The model under review builds one solid part; all positions refer to its coordinate system, in mm. A direction names the side the tool comes from. Coordinates: 2 decimals unless noted, no trailing zeros. Write each loop counter-clockwise with the first axis right and the second up, starting at its lowest first coordinate (ties: lowest second). Pieces come first, ordered by that corner, then holes. Notation, with made-up numbers: (-2.5, 64.5) - (2.5, 64.5) arc R25 cw to (2.5, 84.5) - close; hole circle Ø1 at (73, 14.25). An arc over 180 degrees is marked (long way). Return JSON: item names as keys, results as strings. Group by question number.
(1) We need section A-A on z = 220.5. State the section outline as (x, y) points.
(2) We need section C-C on x = -3.5. Give the number of separate pieces and of enclosed holes in the cut face, then the cut area to 3 significant figures.
(3) Draft analysis for pull direction Z (two halves, no side actions). For faces 5 (the face through (4.65, 9.8, 213.87)), 6 (the face through (-6, 4, 260.5)), 7 (the face through (-5, 4, 205.5)), state which applies: released by +Z, released by -Z, zero draft, split by the parting line, or undercut.
(4) To check wall thickness, follow L1, parallel to X at y = 1, z = 208.5; L2, parallel to Z at x = -3.5, y = 2.5; L3, parallel to X at y = 5, z = 223.5. State the ranges of each line that lie inside material, in increasing order. Write a range as from..to.
(5) Tool access review of faces 1 (the face through (-15.93, 9.8, 213.85)), 2 (the face through (4.65, -2.8, 213.87)), 3 (the face through (10, 4, 253)), 4 (the face through (-16.3, 4, 233)): name each direction out of +Z, -Z, +X, -X, +Y, -Y from which nothing blocks a thin tool from reaching the whole face with its end or side.
(6) We need section B-B on y = 5.75. State the section outline as (x, z) points.
(7) We need section D-D on x = -10.5. State the section outline as (y, z) points, then the cut area to 3 significant figures.
(8) For pin 1 Ø1 at (y, z) = (0, 246) entering from +X; pin 2 Ø3.5 at (y, z) = (4, 255) entering from +X; pin 3 Ø2.5 at (x, z) = (-3.5, 208.5) entering from +Y; pin 4 Ø5 at (x, z) = (-16.5, 257.5) entering from +Y, all flat-tipped, find the tip position at first contact; note any pin that passes through.
```python
from build123d import *

# Parameters (mm, degrees)
SKETCH151_R     = 1.6
PAD085_DEPTH    = 13
CHAMFER055_SIZE = 1
FILLET050_R     = 5
CHAMFER061_SIZE = 0.4


with BuildPart() as part:
    # Sketch151 → Pad085 (new body)
    with BuildSketch(Plane.XZ):
        with BuildLine():
            Line((-11.3, 27.5), (20, 27.5))
            Line((20, 11.599342), (20, 27.5))
            ThreePointArc((20, -3.599342), (25.5, 4), (20, 11.599342))
            Line((20, -27.5), (20, -3.599342))
            Line((20, -27.5), (-11.3, -27.5))
            Line((-11.3, -27.5), (-11.3, 27.5))
        make_face()
        with Locations((-6.5, 24.5)):
            Circle(SKETCH151_R, mode=Mode.SUBTRACT)
        with Locations((6.5, 24.5)):
            Circle(SKETCH151_R, mode=Mode.SUBTRACT)
        with Locations((-6.5, -24.5)):
            Circle(SKETCH151_R, mode=Mode.SUBTRACT)
        with Locations((6.5, -24.5)):
            Circle(SKETCH151_R, mode=Mode.SUBTRACT)
        with BuildLine():
            Line((-6.3, 19.5), (15, 19.5))
            Line((15, 8.330127), (15, 19.5))
            ThreePointArc((15, -0.330127), (22.5, 4), (15, 8.330127))
            Line((15, -19.5), (15, -0.330127))
            Line((15, -19.5), (-6.3, -19.5))
            Line((-6.3, -19.5), (-6.3, 19.5))
        make_face(mode=Mode.SUBTRACT)
    extrude(amount=PAD085_DEPTH)

    # Chamfer055
    chamfer055_edges = [part.edges().sort_by_distance(p)[0] for p in [
        (-11.3, -6.5, -27.5),
        (20, -6.5, -27.5),
        (-11.3, -6.5, 27.5),
        (20, -6.5, 27.5),
        (-6.3, -6.5, 19.5),
        (-6.3, -6.5, -19.5),
        (15, -6.5, -19.5),
        (15, -6.5, 19.5),
    ]]
    chamfer(chamfer055_edges, length=CHAMFER055_SIZE)

    # Fillet050
    fillet050_edges = [part.edges().sort_by_distance(p)[0] for p in [
        (15, -6.5, 8.330127),
        (15, -6.5, -0.330127),
        (20, -6.5, -3.599342),
        (20, -6.5, 11.599342),
    ]]
    fillet(fillet050_edges, radius=FILLET050_R)

    # Chamfer061
    chamfer061_edges = [part.edges().sort_by_distance(p)[0] for p in [
        (16.047153, -13, 10.620596),
        (16.047153, 0, 10.620596),
        (14.5, -13, 19),
        (4.35, -13, 19.5),
        (-5.8, -13, 19),
        (-6.3, -13, 0),
        (-5.8, -13, -19),
        (4.35, -13, -19.5),
        (14.5, -13, -19),
        (14.5, 0, -19),
        (4.35, 0, -19.5),
        (-5.8, 0, -19),
        (-6.3, 0, 0),
        (-5.8, 0, 19),
        (4.35, 0, 19.5),
        (14.5, 0, 19),
        (-11.3, -13, 0),
        (-10.8, -13, 27),
        (4.35, -13, 27.5),
        (19.5, -13, 27),
        (20, -13, 20.55919),
        (19.5, -13, -27),
        (4.35, -13, -27.5),
        (-10.8, -13, -27),
        (-11.3, 0, 0),
        (-10.8, 0, 27),
        (4.35, 0, 27.5),
        (20, 0, 20.55919),
        (19.5, 0, 27),
        (19.5, 0, -27),
        (-10.8, 0, -27),
        (4.35, 0, -27.5),
        (-8.1, 0, 24.5),
        (4.9, 0, 24.5),
        (4.9, -13, 24.5),
        (-8.1, -13, 24.5),
        (4.9, 0, -24.5),
        (-8.1, 0, -24.5),
        (-8.1, -13, -24.5),
        (4.9, -13, -24.5),
    ]]
    chamfer(chamfer061_edges, length=CHAMFER061_SIZE)


with BuildPart() as part_1:
    # Body073 placement: moved
    add(part.part.moved(Location((-10, 10, 233))))


solid = part_1.part
```
Ans:
{
 "1": {"outline": "(-21.3, -2.6) - (-20.9, -3) - (-16.7, -3) - (-16.3, -2.6) - (-16.3, 9.6) - (-16.7, 10) - (-20.9, 10) - (-21.3, 9.6) - close; (5, -2.6) - (5.4, -3) - (9.6, -3) - (10, -2.6) - (10, 9.6) - (9.6, 10) - (5.4, 10) - (5, 9.6) - close"},
 "2": {"separate pieces": "4", "enclosed holes": "0", "area": "124 mm²"},
 "3": {"face 5": "undercut", "face 6": "released by +Z", "face 7": "released by -Z"},
 "4": {"L1": "-21.3..-18.1, -14.9..-5.1, -1.9..10", "L2": "205.5..206.9, 210.1..213.5, 252.5..255.9, 259.1..260.5", "L3": "-21.3..-16.3, 5..10"},
 "5": {"face 1": "+Y", "face 2": "-Y", "face 3": "+Z, +X, +Y, -Y", "face 4": "+Y, -Y"},
 "6": {"outline": "(-21.3, 206.5) - (-20.3, 205.5) - (9, 205.5) - (10, 206.5) - (10, 226.38) arc R5 cw to (12.12, 230.47) arc R8 ccw to (12.12, 243.53) arc R5 cw to (10, 247.62) - (10, 259.5) - (9, 260.5) - (-20.3, 260.5) - (-21.3, 259.5) - close; hole circle Ø3.2 at (-16.5, 208.5); hole circle Ø3.2 at (-16.5, 257.5); hole (-16.3, 214.5) - (-15.3, 213.5) - (4, 213.5) - (5, 214.5) - (5, 227.32) arc R5 cw to (8.75, 232.16) arc R5 ccw to (8.75, 241.84) arc R5 cw to (5, 246.68) - (5, 251.5) - (4, 252.5) - (-15.3, 252.5) - (-16.3, 251.5) - close; hole circle Ø3.2 at (-3.5, 208.5); hole circle Ø3.2 at (-3.5, 257.5)"},
 "7": {"outline": "(-3, 205.9) - (-2.6, 205.5) - (9.6, 205.5) - (10, 205.9) - (10, 213.1) - (9.6, 213.5) - (-2.6, 213.5) - (-3, 213.1) - close; (-3, 252.9) - (-2.6, 252.5) - (9.6, 252.5) - (10, 252.9) - (10, 260.1) - (9.6, 260.5) - (-2.6, 260.5) - (-3, 260.1) - close", "area": "207 mm²"},
 "8": {"pin 1": "x = 10.47", "pin 2": "x = 10", "pin 3": "through", "pin 4": "y = 10"}
}
